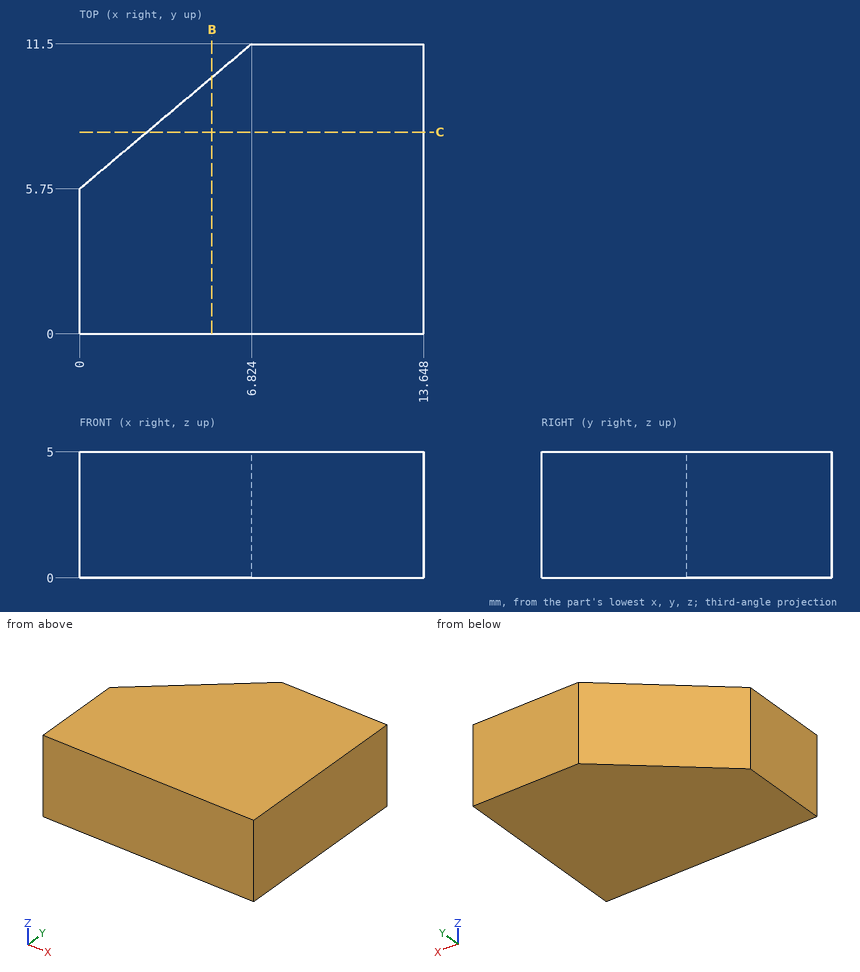
Source: three-view drawing plus pictorial views. Frame: mm from the lowest corner of the part. Coordinates: 2 decimals unless noted, no trailing zeros. Loops run counter-clockwise (first coordinate to the right, second up) from the corner with the lowest first, then second, coordinate; pieces in that order, holes last. Notation, with made-up numbers: (19.5, 35) - (26.5, 35) arc R23 ccw to (26.5, 43) - close; hole circle Ø8 at (-23, -4). An arc over 180 degrees is marked (long way). Answer in a Markdown table with one row per item. Add a question column.
Item 1: Contact query for a flat-ended pin moving along its axis: P1, Ø2, axis at x = 4.5, y = 5, coming from the -Z side. Output: stop coordinate, or through.
Item 2: Line query: line 1 along Y through (x, z) = (6, 4.25) (1 decimal); line 2 along Y through (x, z) = (4.75, 1.5); line 3 along X through (y, z) = (8, 0.6). Output: solid intervals per line, ascending. Write a range as [from, to].
Item 3: Section query B-B on x = 5.25. Return the cut outline in (y, z).
Item 4: Section query C-C on y = 8. Return the cut outline in (x, z), then the cut area to 3 significant figures.
Recorded:
| question | item | result |
|---|---|---|
| 1 | P1 | z = 0 |
| 2 | line 1 | [0, 10.8] |
| 2 | line 2 | [0, 9.75] |
| 2 | line 3 | [2.67, 13.65] |
| 3 | outline | (0, 0) - (10.17, 0) - (10.17, 5) - (0, 5) - close |
| 4 | outline | (2.67, 0) - (13.65, 0) - (13.65, 5) - (2.67, 5) - close |
| 4 | area | 54.9 mm^2 |
